Autodesk Fusion 360 part; units mm, degrees
sketch "Sketch1" plane through (0, 0, 0) normal (0, 1, 0) x (1, 0, 0)
  line L0 (0, 0) -> (83.4, 0)
  line L1 (83.4, 0) -> (83.4, 19.8)
  line L2 (83.4, 19.8) -> (0, 19.8)
  line L3 (0, 19.8) -> (0, 0)
  circle A0 centre (6.5, 9.9) radius 5
  circle A1 centre (76.9, 9.9) radius 5
  line L4 (16.7, 12.3) -> (66.7, 12.3)
  line L5 (66.7, 12.3) -> (66.7, 7.5)
  line L6 (66.7, 7.5) -> (16.7, 7.5)
  line L7 (16.7, 7.5) -> (16.7, 12.3)
  circle A2 centre (76.9, 9.9) radius 2.8
  circle A3 centre (6.5, 9.9) radius 2.8
  point P0 (66.7, 9.9)
  point P1 (83.4, 9.9)
  point P2 (41.7, 12.3)
  point P3 (41.7, 19.8)
  dimension "d1" = 83.4
  dimension "d2" = 19.8
  dimension "d3" = 10
  dimension "d4" = 6.5
  dimension "d5" = 10
  dimension "d6" = 6.5
  dimension "d7" = 50
  dimension "d9" = 4.8
  dimension "d18" = 5.6
  dimension "d19" = 5.6
extrude "Extrude1" add sketch "Sketch1" along normal blind 17.8 contours L4 L5 L6 L7 makes body 1
extrude "Extrude2" add sketch "Sketch1" along normal blind 3.8 separate body contours L0 L1 L2 L3 makes body 2
extrude "Extrude3" add sketch "Sketch1" along normal blind 3.8 separate body contours A0 | A1 | A2 | A3 makes body 3 at (81.8938, 1.2667, -9.6508) makes body 4 at (11.4752, 2.5333, -9.4022)
extrude "Extrude4" cut sketch "Sketch1" along normal blind 3.8 draft 30 contours A2 | A3 bodies 3 4
combine "Combine1" operation add target body 2 tool bodies 1
combine "Combine2" operation add target body 2 tool bodies 3 4
fillet "Fillet1" radius 0.6 12 edges at (66.7, 10.8, -12.3) (66.7, 10.8, -7.5) (41.7, 17.8, -12.3) (83.4, 3.8, -9.9) (41.7, 3.8, -19.8) (41.7, 3.8, 0) (66.7, 17.8, -9.9) (16.7, 17.8, -9.9) (0, 3.8, -9.9) (41.7, 17.8, -7.5) (16.7, 10.8, -7.5) (16.7, 10.8, -12.3) on bodies 2
fillet "Fillet2" radius 2.5 8 edges at (66.5243, 3.8, -12.1243) (66.7, 3.8, -9.9) (66.5243, 3.8, -7.6757) (41.7, 3.8, -7.5) (16.8757, 3.8, -7.6757) (16.7, 3.8, -9.9) (16.8757, 3.8, -12.1243) (41.7, 3.8, -12.3) on bodies 2
equation "d3 = screw_top_opening_width"
equation "d5 = screw_top_opening_width"
equation "plate_height = 3.8 mm"
equation "d14 = 14 mm + plate_height"
equation "d16 = plate_height"
equation "d18 = screw_bottom_opening_width"
equation "d19 = screw_bottom_opening_width"
equation "screw_top_opening_width = 10 mm"
equation "screw_bottom_opening_width = 5.6 mm"
equation "d22 = plate_height"
equation "d24 = plate_height"
equation "screw_taper_angle = 30 deg"
equation "outside_fillet_radiu = 0.6 mm"
equation "d29 = outside_fillet_radiu"
equation "inside_fillet_radius = 2.5 mm"
equation "d32 = inside_fillet_radius"
Could you check a few things on this model? Use its own coordinates, in mm. A direction names the side the tool comes from. Round coordinates to 2 decimals unless told otherwise and drop trailing zeros. Write each loop counter-clockwise with the first axis right and the second up, starting at its lowest first coordinate (ties: lowest second). Pieces come first, ordered by that corner, then holes. Notation, with made-up numbers: (87, 48.5) - (122, 48.5) arc R8 ccw to (122, 63.5) - close; hole circle Ø9 at (55.25, 41). An arc over 180 degrees is marked (long way). Use a Markdown table: item, result.
Q1. For faces 1 (the flat face through (66.7, 12, -10)), 2 (the flat face through (16.7, 12, -10)), 3 (the flat face through (41, 2, 0)), which set-ups out of +Z, -Z, +X, -X, +Y, -Y let a thin tool reach every point of the face, with its end or its side?
Output values:
| item | result |
|---|---|
| face 1 | +Z, -Z, +X, +Y |
| face 2 | +Z, -Z, -X, +Y |
| face 3 | +Z, +X, -X, +Y, -Y |
Q2. Thinking about a two-plate mould opening in Z: for faces 4 (the flat face through (41, 3.8, -16)), 5 (the flat face through (41, 12, -12.3)), 6 (the conical face through (3.566, 0.238, -10.029)), 7 (the flat face through (42, 12, -7.5)), which applies, released by +Z, released by -Z, zero draft, split by the parting line, or undercut?
Output values:
| item | result |
|---|---|
| face 4 | zero draft |
| face 5 | released by -Z |
| face 6 | undercut |
| face 7 | released by +Z |
Q3. Please list where these lines run through material, in increasing order: L1, parallel to X at y = 2.5, z = -13; L2, parallel to X at y = 1.25, z = -12; L3, parallel to Z at x = 24.5, y = 16.5.
Output values:
| item | result |
|---|---|
| L1 | 0 to 3.6, 9.4 to 74, 79.8 to 83.4 |
| L2 | 0 to 3.67, 9.33 to 74.07, 79.73 to 83.4 |
| L3 | -12.3 to -7.5 |
Q4. I want a section at B-B (z = -9.9). List the corners of the cut face in (x, y) for me, plus the area to 3 significant figures.
Output values:
| item | result |
|---|---|
| outline | (0, 0) - (3.7, 0) - (1.51, 3.8) - (0.6, 3.8) arc R0.6 ccw to (0, 3.2) - close; (9.3, 0) - (74.1, 0) - (71.91, 3.8) - (69.2, 3.8) arc R2.5 cw to (66.7, 6.3) - (66.7, 17.2) arc R0.6 ccw to (66.1, 17.8) - (17.3, 17.8) arc R0.6 ccw to (16.7, 17.2) - (16.7, 6.3) arc R2.5 cw to (14.2, 3.8) - (11.49, 3.8) - close; (79.7, 0) - (83.4, 0) - (83.4, 3.2) arc R0.6 ccw to (82.8, 3.8) - (81.89, 3.8) - close |
| area | 960 mm2 |
Q5. I want a section at A-A (x = 6.5). List the corners of the cut face in (y, z) for me.
Output values:
| item | result |
|---|---|
| outline | (0, -19.8) - (3.2, -19.8) arc R0.6 ccw to (3.8, -19.2) - (3.8, -14.89) - (0, -12.7) - close; (0, -7.1) - (3.8, -4.91) - (3.8, -0.6) arc R0.6 ccw to (3.2, 0) - (0, 0) - close |
Q6. I want a section at C-C (y = 12.25). List the corners of the cut face in (x, z) for me, plus the area to 3 significant figures.
Output values:
| item | result |
|---|---|
| outline | (16.7, -11.7) arc R0.6 ccw to (17.3, -12.3) - (66.1, -12.3) arc R0.6 ccw to (66.7, -11.7) - (66.7, -8.1) arc R0.6 ccw to (66.1, -7.5) - (17.3, -7.5) arc R0.6 ccw to (16.7, -8.1) - close |
| area | 240 mm2 |
Q7. I want a section at D-D (x = 49). List the corners of the cut face in (y, z) for me, plus the area to 3 significant figures.
Output values:
| item | result |
|---|---|
| outline | (0, -19.8) - (3.2, -19.8) arc R0.6 ccw to (3.8, -19.2) - (3.8, -14.8) arc R2.5 cw to (6.3, -12.3) - (17.2, -12.3) arc R0.6 ccw to (17.8, -11.7) - (17.8, -8.1) arc R0.6 ccw to (17.2, -7.5) - (6.3, -7.5) arc R2.5 cw to (3.8, -5) - (3.8, -0.6) arc R0.6 ccw to (3.2, 0) - (0, 0) - close |
| area | 145 mm2 |
Q8. For pin 1 (8.5 mm diameter, centred on x = 51, y = 13.5, fed in from -Z); pin 2 (1.8 mm diameter, centred on y = 11, z = -11, fed in from -X); pin 3 (4 mm diameter, centred on y = 10, z = -10, fed in from +X), each with a flat end and sliding along its axis, tell me the tip position at first contact or that it passes through.
Output values:
| item | result |
|---|---|
| pin 1 | z = -12.3 |
| pin 2 | x = 16.7 |
| pin 3 | x = 66.7 |
